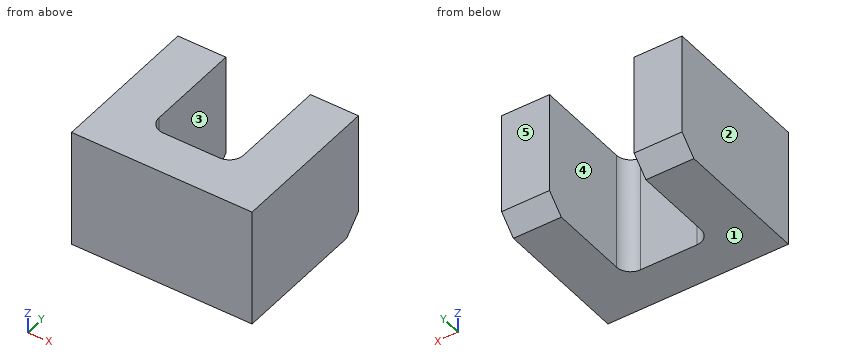
```python
from build123d import *

# Parameters (mm, degrees)
SKETCH1_W           = 6.4
SKETCH1_H           = 4.2
BOSS_EXTRUDE1_DEPTH = 5.4
SKETCH2_W           = 3
SKETCH2_H           = 4.2
CUT_EXTRUDE1_DEPTH  = 3.9
FILLET1_R           = 0.5
CHAMFER1_SIZE       = 0.6


with BuildPart() as part:
    # Sketch1 → Boss-Extrude1 (new body)
    with BuildSketch(Plane(origin=(0, 0, 0), x_dir=(1, 0, 0), z_dir=(0, 1, 0))):
        Rectangle(SKETCH1_W, SKETCH1_H)
    extrude(amount=BOSS_EXTRUDE1_DEPTH)

    # Sketch2 → Cut-Extrude1 (cut)
    with BuildSketch(Plane(origin=(0, 5.4, 0), x_dir=(1, 0, 0), z_dir=(0, 1, 0))):
        Rectangle(SKETCH2_W, SKETCH2_H)
    extrude(amount=-CUT_EXTRUDE1_DEPTH, mode=Mode.SUBTRACT)

    # Fillet1
    fillet1_edges = [part.edges().sort_by_distance(p)[0] for p in [
        (-1.5, 1.5, 0),
        (1.5, 1.5, 0),
    ]]
    fillet(fillet1_edges, radius=FILLET1_R)

    # Chamfer1
    chamfer1_edges = [part.edges().sort_by_distance(p)[0] for p in [
        (2.35, 5.4, -2.1),
        (-2.35, 5.4, -2.1),
    ]]
    chamfer(chamfer1_edges, length=CHAMFER1_SIZE)


solid = part.part
```
Verification items for the finished model (mm, model axes). Face numbers are marked on the shaded views. A direction names the side the tool comes from. Coordinates: 2 decimals unless noted, no trailing zeros. Order: outer loops, then holes, each group sorted by start corner. A loop starts at its lowest first (then second) coordinate and runs counter-clockwise, first axis right, second up. Notation, with made-up numbers: (26.5, -14.75) -> (62.5, -14.75) arc R25 cw to (62.5, 15.25) -> close; hole circle Ø2 at (25.5, -13.5). An arc over 180 degrees is marked (long way). Put each result on its own line as item: value. Start each with the question number.
1) Go/stop test with a flat-tipped pin: pin 1 (2 mm diameter, centred on x = 0, z = -0.5, fed in from +Y). Record where the tip stops, or that it passes through.
2) Material ranges on L1, parallel to X at y = 2.2, z = -1.15; L2, parallel to Y at x = 0.5, z = 0.05; L3, parallel to X at y = 1.75, z = -0.8, recorded low to high.
3) Cross-section at A-A (y = 3.6). Enter the section's corners in (x, z).
4) Cross-section at C-C (y = 4.9). Enter the section's corners in (x, z).
5) Cross-section at B-B (z = 1.05). Enter the section's corners in (x, y), plus the area to 3 significant figures.
6) Tool access check on the marked faces 4 and 5. Record the directions out of +Z, -Z, +X, -X, +Y, -Y that give a thin tool (end or side, any length) a straight path to the whole face; none if there is none.
7) Cross-section at D-D (x = -1.25). Enter the section's corners in (y, z), plus the area to 3 significant figures.
8) Release check for a two-part mould opening along X. For the marked faces 1, 2 and 3 record: pulls with the +X half, pulls with the -X half, needs draft (parallel to the pull), parting line crosses it, or undercut.
Geometry check:
1. pin 1: stops at y = 1.5
2. L1: x = -3.2 to -1.5, 1.5 to 3.2
2. L2: y = 0 to 1.5
2. L3: x = -3.2 to -1.43, 1.43 to 3.2
3. outline: (-3.2, -2.1) -> (-1.5, -2.1) -> (-1.5, 2.1) -> (-3.2, 2.1) -> close; (1.5, -2.1) -> (3.2, -2.1) -> (3.2, 2.1) -> (1.5, 2.1) -> close
4. outline: (-3.2, -2) -> (-1.5, -2) -> (-1.5, 2.1) -> (-3.2, 2.1) -> close; (1.5, -2) -> (3.2, -2) -> (3.2, 2.1) -> (1.5, 2.1) -> close
5. outline: (-3.2, 0) -> (3.2, 0) -> (3.2, 5.4) -> (1.5, 5.4) -> (1.5, 2) arc R0.5 cw to (1, 1.5) -> (-1, 1.5) arc R0.5 cw to (-1.5, 2) -> (-1.5, 5.4) -> (-3.2, 5.4) -> close
5. area: 23.0 mm^2
6. face 4: +Z, -Z, +Y
6. face 5: +Z, -Z, +X, -X, +Y
7. outline: (0, -2.1) -> (1.57, -2.1) -> (1.57, 2.1) -> (0, 2.1) -> close
7. area: 6.58 mm^2
8. face 1: needs draft
8. face 2: pulls with the -X half
8. face 3: undercut
